from build123d import *

# Parameters (mm, degrees)
SKETCH1_W           = 25.4
SKETCH1_H           = 25.4
SKETCH1_W_2         = 22.225
SKETCH1_H_2         = 22.225
BOSS_EXTRUDE1_DEPTH = 292.1
SKETCH2_R           = 2.5527
CUT_EXTRUDE1_DEPTH  = 294.477188211
SKETCH3_R           = 2.5527
CUT_EXTRUDE2_DEPTH  = 294.477188211


with BuildPart() as part:
    # Sketch1 → Boss-Extrude1 (new body)
    with BuildSketch(Plane.XY):
        Rectangle(SKETCH1_W, SKETCH1_H)
        Rectangle(SKETCH1_W_2, SKETCH1_H_2, mode=Mode.SUBTRACT)
    extrude(amount=BOSS_EXTRUDE1_DEPTH)

    # Sketch2 → Cut-Extrude1 (cut, through all)
    with BuildSketch(Plane(origin=(0, 12.7, 0), x_dir=(1, 0, 0), z_dir=(0, 1, 0))):
        Circle(SKETCH2_R)
        with Locations(Location((0, -12.7, 0), (0, 0, 270))):
            Circle(SKETCH2_R)
        with Locations(Location((0, -25.4, 0), (0, 0, 270))):
            Circle(SKETCH2_R)
        with Locations(Location((0, -38.1, 0), (0, 0, 270))):
            Circle(SKETCH2_R)
        with Locations(Location((0, -50.8, 0), (0, 0, 270))):
            Circle(SKETCH2_R)
        with Locations(Location((0, -63.5, 0), (0, 0, 270))):
            Circle(SKETCH2_R)
        with Locations(Location((0, -76.2, 0), (0, 0, 270))):
            Circle(SKETCH2_R)
        with Locations(Location((0, -88.9, 0), (0, 0, 270))):
            Circle(SKETCH2_R)
        with Locations(Location((0, -101.6, 0), (0, 0, 270))):
            Circle(SKETCH2_R)
        with Locations(Location((0, -114.3, 0), (0, 0, 270))):
            Circle(SKETCH2_R)
        with Locations(Location((0, -127, 0), (0, 0, 270))):
            Circle(SKETCH2_R)
        with Locations(Location((0, -139.7, 0), (0, 0, 270))):
            Circle(SKETCH2_R)
        with Locations(Location((0, -152.4, 0), (0, 0, 270))):
            Circle(SKETCH2_R)
        with Locations(Location((0, -165.1, 0), (0, 0, 270))):
            Circle(SKETCH2_R)
        with Locations(Location((0, -177.8, 0), (0, 0, 270))):
            Circle(SKETCH2_R)
        with Locations(Location((0, -190.5, 0), (0, 0, 270))):
            Circle(SKETCH2_R)
        with Locations(Location((0, -203.2, 0), (0, 0, 270))):
            Circle(SKETCH2_R)
        with Locations(Location((0, -215.9, 0), (0, 0, 270))):
            Circle(SKETCH2_R)
        with Locations(Location((0, -228.6, 0), (0, 0, 270))):
            Circle(SKETCH2_R)
        with Locations(Location((0, -241.3, 0), (0, 0, 270))):
            Circle(SKETCH2_R)
        with Locations(Location((0, -254, 0), (0, 0, 270))):
            Circle(SKETCH2_R)
        with Locations(Location((0, -266.7, 0), (0, 0, 270))):
            Circle(SKETCH2_R)
        with Locations(Location((0, -279.4, 0), (0, 0, 270))):
            Circle(SKETCH2_R)
        with Locations((0, -292.1)):
            Circle(SKETCH2_R)
        with Locations((0, -304.8)):
            Circle(SKETCH2_R)
        with Locations((0, -317.5)):
            Circle(SKETCH2_R)
    extrude(amount=-CUT_EXTRUDE1_DEPTH, mode=Mode.SUBTRACT)

    # Sketch3 → Cut-Extrude2 (cut, through all)
    with BuildSketch(Plane(origin=(12.7, 0, 0), x_dir=(0, 0, -1), z_dir=(1, 0, 0))):
        Circle(SKETCH3_R)
        with Locations(Location((-12.7, 0, 0), (0, 0, 90))):
            Circle(SKETCH3_R)
        with Locations(Location((-25.4, 0, 0), (0, 0, 90))):
            Circle(SKETCH3_R)
        with Locations(Location((-38.1, 0, 0), (0, 0, 90))):
            Circle(SKETCH3_R)
        with Locations(Location((-50.8, 0, 0), (0, 0, 90))):
            Circle(SKETCH3_R)
        with Locations(Location((-63.5, 0, 0), (0, 0, 90))):
            Circle(SKETCH3_R)
        with Locations(Location((-76.2, 0, 0), (0, 0, 90))):
            Circle(SKETCH3_R)
        with Locations(Location((-88.9, 0, 0), (0, 0, 90))):
            Circle(SKETCH3_R)
        with Locations(Location((-101.6, 0, 0), (0, 0, 90))):
            Circle(SKETCH3_R)
        with Locations(Location((-114.3, 0, 0), (0, 0, 90))):
            Circle(SKETCH3_R)
        with Locations(Location((-127, 0, 0), (0, 0, 90))):
            Circle(SKETCH3_R)
        with Locations(Location((-139.7, 0, 0), (0, 0, 90))):
            Circle(SKETCH3_R)
        with Locations(Location((-152.4, 0, 0), (0, 0, 90))):
            Circle(SKETCH3_R)
        with Locations(Location((-165.1, 0, 0), (0, 0, 90))):
            Circle(SKETCH3_R)
        with Locations(Location((-177.8, 0, 0), (0, 0, 90))):
            Circle(SKETCH3_R)
        with Locations(Location((-190.5, 0, 0), (0, 0, 90))):
            Circle(SKETCH3_R)
        with Locations(Location((-203.2, 0, 0), (0, 0, 90))):
            Circle(SKETCH3_R)
        with Locations(Location((-215.9, 0, 0), (0, 0, 90))):
            Circle(SKETCH3_R)
        with Locations(Location((-228.6, 0, 0), (0, 0, 90))):
            Circle(SKETCH3_R)
        with Locations(Location((-241.3, 0, 0), (0, 0, 90))):
            Circle(SKETCH3_R)
        with Locations(Location((-254, 0, 0), (0, 0, 90))):
            Circle(SKETCH3_R)
        with Locations(Location((-266.7, 0, 0), (0, 0, 90))):
            Circle(SKETCH3_R)
        with Locations(Location((-279.4, 0, 0), (0, 0, 90))):
            Circle(SKETCH3_R)
        with Locations((-292.1, 0)):
            Circle(SKETCH3_R)
        with Locations((-304.8, 0)):
            Circle(SKETCH3_R)
        with Locations((-317.5, 0)):
            Circle(SKETCH3_R)
    extrude(amount=-CUT_EXTRUDE2_DEPTH, mode=Mode.SUBTRACT)


solid = part.part
The model under review builds one solid part; all positions refer to its coordinate system, in mm. A direction names the side the tool comes from. Round coordinates to 2 decimals unless told otherwise and drop trailing zeros. Write each loop counter-clockwise with the first axis right and the second up, starting at its lowest first coordinate (ties: lowest second). Pieces come first, ordered by that corner, then holes. Notation, with made-up numbers: M 31.25,24 L 40.25,24 A20 cw 40.25,50 Z; hole C 72,73.25 d3. An arc over 180 degrees is marked long. Use a Markdown table: item, result. Add a question column.
Q1. We need section A-A, the plane x = -6.75. State the section outline as (y, z) points, plus the area to 3 significant figures.
Q2. To check wall thickness, follow line 1 (X direction, y = -10.75, z = 149); line 2 (X direction, y = 11.85, z = 228.6). State the ranges of each line that lie inside material, in increasing order.
Q3. We need section B-B, the plane z = 241.3. State the section outline as (x, y) points, plus the area to 3 significant figures.
Q4. Insertion check: pin 1 (8 mm diameter, centred on y = 0, z = 228.6, fed in from +X). The pin has a flat end and moves straight along its axis. Give the tip position at first contact, or say it passes through.
Q5. Machinability: for faces 3 (the face through (11.112, 0, 144)), 4 (the face through (0.11, 11.92, 251.45)), which of the approach directions +Z, -Z, +X, -X, +Y, -Y give a long, thin tool a straight path to every point of the face, cutting with its end or side? Answer none if there is none.
Q6. The part is to be moulded in two halves that separate along X. For faces 1 (the face through (-11.895, -0.553, 226.108)), 2 (the face through (0.767, -11.895, 15.135)), say which applies: pulls with the +X half, pulls with the -X half, needs draft (parallel to the pull), parting line crosses it, or undercut.
Q7. We need section D-D, the plane z = 94.5. State the section outline as (x, y) points.
Findings below:
| question | item | result |
|---|---|---|
| 1 | outline | M -12.7,0 L -11.11,0 L -11.11,292.1 L -12.7,292.1 Z; M 11.11,0 L 12.7,0 L 12.7,292.1 L 11.11,292.1 Z |
| 1 | area | 927 mm² |
| 2 | line 1 | x = -12.7 to -11.11, 11.11 to 12.7 |
| 2 | line 2 | x = -12.7 to -2.55, 2.55 to 12.7 |
| 3 | outline | M -12.7,-12.7 L -2.55,-12.7 L -2.55,-11.11 L -11.11,-11.11 L -11.11,-2.55 L -12.7,-2.55 Z; M -12.7,2.55 L -11.11,2.55 L -11.11,11.11 L -2.55,11.11 L -2.55,12.7 L -12.7,12.7 Z; M 2.55,-12.7 L 12.7,-12.7 L 12.7,-2.55 L 11.11,-2.55 L 11.11,-11.11 L 2.55,-11.11 Z; M 2.55,11.11 L 11.11,11.11 L 11.11,2.55 L 12.7,2.55 L 12.7,12.7 L 2.55,12.7 Z |
| 3 | area | 119 mm² |
| 4 | pin 1 | stops at x = 12.7 |
| 5 | face 3 | +Z, -Z |
| 5 | face 4 | +Y, -Y |
| 6 | face 1 | needs draft |
| 6 | face 2 | undercut |
| 7 | outline | M -12.7,-12.7 L 12.7,-12.7 L 12.7,12.7 L -12.7,12.7 Z; hole M -11.11,-11.11 L 11.11,-11.11 L 11.11,11.11 L -11.11,11.11 Z |
